The listing builds one solid part. Answer for the finished solid, in the listing's coordinates (mm). Face numbers are marked on the shaded views. Round coordinates to 2 decimals unless told otherwise and drop trailing zeros. Loops run counter-clockwise (first coordinate to the right, second up) from the corner with the lowest first, then second, coordinate; pieces in that order, holes last. Notation, with made-up numbers: (23, -28) -> (52, -28) arc R15 ccw to (52, 1) -> close; hole circle Ø11 at (79.5, -28.75). An arc over 180 degrees is marked (long way). Write each question's results on one line, items separated by ' | '. Start each with the question number.
(1) Determine the mould class of the marked faces 1, 2, 3 and 4 for opening direction X: released by +X, released by -X, zero draft, split by the parting line, or undercut.
(2) The part is cut by section C-C (y = 13.5). Determine the outline of the cut face in (x, z), plus the area to 3 significant figures.
(3) Straight lines are drawn through the part: probe 1 along X at (y, z) = (6, 0.75); probe 2 along X at (y, z) = (-6.5, 6.5); probe 3 along Y at (x, z) = (-5, 4.75). For each, find the intervals that lie inside material, in ascending order.
(4) The part is cut by section B-B (z = 2.5). Determine the outline of the cut face in (x, y), plus the area to 3 significant figures.
(5) The part is cut by section D-D (y = -11). Determine the outline of the cut face in (x, z).
(6) Flat-ended cylindrical pins translate along their axes: pin 1 (1 mm diameter, centred on x = 6.5, z = 3, fed in from -Y); pin 2 (3 mm diameter, centred on x = 9.5, z = 6, fed in from +Y); pin 3 (1 mm diameter, centred on x = -7, z = 6, fed in from -Y). Find the tip coordinate at first contact, or state that the pin passes through.
(7) The part is cut by section A-A (y = 0). Determine the outline of the cut face in (x, z), plus the area to 3 significant figures.
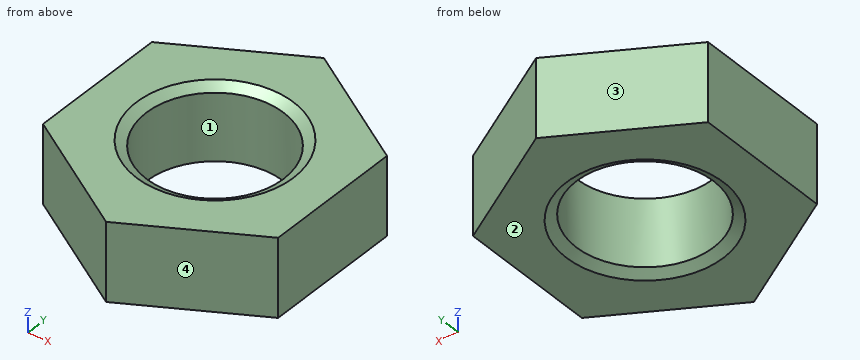
```python
from build123d import *

# Parameters (mm, degrees)
SKETCH001_R  = 18
POCKET_DEPTH = 10


with BuildPart() as part:
    # Sketch → Revolution (revolve)
    with BuildSketch(Plane.XZ):
        Polygon((10, 0), (8.75, 0.721688), (8.75, 9.278312), (10, 10), (18, 10), (18, 0), align=None)
    revolve(axis=Axis((0, 0, 0), (0, 0, 1)))

    # Sketch001 → Pocket (cut)
    with BuildSketch(Plane(origin=(0, 0, 10), x_dir=(-1, 0, 0), z_dir=(0, 0, 1))):
        Circle(SKETCH001_R)
        Polygon((-15, 8.660254), (-15, -8.660254), (0, -17.320508), (15, -8.660254), (15, 8.660254), (0, 17.320508), align=None, mode=Mode.SUBTRACT)
    extrude(amount=-POCKET_DEPTH, mode=Mode.SUBTRACT)


solid = part.part
```
Checked values:
1) face 1: undercut | face 2: zero draft | face 3: released by -X | face 4: released by +X
2) outline: (-6.62, 0) -> (6.62, 0) -> (6.62, 10) -> (-6.62, 10) -> close | area: 132 mm2
3) probe 1: x = -15 to -6.37, 6.37 to 15 | probe 2: x = -15 to -5.86, 5.86 to 15 | probe 3: y = -14.43 to -7.18, 7.18 to 14.43
4) outline: (-15, -8.66) -> (0, -17.32) -> (15, -8.66) -> (15, 8.66) -> (0, 17.32) -> (-15, 8.66) -> close; hole circle Ø17.5 at (0, 0) | area: 539 mm2
5) outline: (-10.95, 0) -> (10.95, 0) -> (10.95, 10) -> (-10.95, 10) -> close
6) pin 1: stops at y = -13.86 | pin 2: stops at y = 12.7 | pin 3: stops at y = -13.57
7) outline: (-15, 0) -> (-10, 0) -> (-8.75, 0.72) -> (-8.75, 9.28) -> (-10, 10) -> (-15, 10) -> close; (8.75, 0.72) -> (10, 0) -> (15, 0) -> (15, 10) -> (10, 10) -> (8.75, 9.28) -> close | area: 123 mm2
